CAD build for the part. Positions are in the model's coordinates, mm. Face numbers are marked on the shaded views. A direction names the side the tool comes from. Round coordinates to 2 decimals unless told otherwise and drop trailing zeros. Write each loop counter-clockwise with the first axis right and the second up, starting at its lowest first coordinate (ties: lowest second). Pieces come first, ordered by that corner, then holes. Notation, with made-up numbers: (2, 37) - (16, 37) arc R31 ccw to (16, 64) - close; hole circle Ø5 at (83.5, 25). An arc over 180 degrees is marked (long way). Use one line per item in the form item = value. Start each with the question number.
Item 1: Band-saw the part on A-A, the plane x = -2. List the corners of the cut face in (y, z), and give its area (3 significant figures).
Item 2: Drill centre lines: L1, parallel to X at y = 7, z = 182; L2, parallel to X at y = 7.5, z = 60.5; L3, parallel to X at y = -22, z = -4. Where is each one in solid material? Low to high.
Item 3: Band-saw the part on C-C, the plane x = 38. List the corners of the cut face in (y, z), and give its area (3 significant figures).
Item 4: Pin check, flat tips, straight feed: pin 1 (7 mm diameter, centred on x = 38, y = -22.5, fed in from -Z); pin 2 (2 mm diameter, centred on x = 27.5, z = 156.5, fed in from -Y); pin 3 (10 mm diameter, centred on x = -24.5, z = 52.5, fed in from +Y); pin 4 (12.5 mm diameter, centred on y = 4, z = 44.5, fed in from -X). Stop position of each tip, or through.
Item 5: Tool access for the marked faces 1, 2, 3 and 4: list every direction of +Z, -Z, +X, -X, +Y, -Y with a clear straight run to the whole face (end or side of a thin tool).
Item 6: Pull direction Z, two halves, no side cores. Call the marked faces 5, 6, 7 and 8: +Z half, -Z half, draft (parallel to the pull), parting line (faces both ways), or undercut.
Item 7: Band-saw the part on B-B, the plane z = 170. List the corners of the cut face in (x, y).
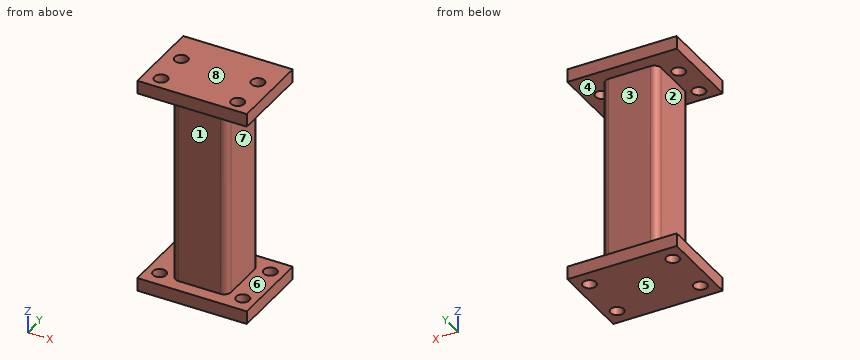
from build123d import *

# Parameters (mm, degrees)
F0_W     = 100
F0_H     = 75
F1_DEPTH = 12
F3_DEPTH = 175.5
F5_W     = 100
F5_H     = 75
F6_DEPTH = 12
F7_D     = 12
F7_DEPTH = 12.001
F9_D     = 12
F9_DEPTH = 12
F9_TIP   = 3.6051637142


with BuildPart() as f1:
    # F0 (on Top) → F1 (new body)
    with BuildSketch(Plane.XY):
        Rectangle(F0_W, F0_H)
    extrude(amount=-F1_DEPTH)

    # F2 (on face) → F3 (join)
    with BuildSketch(Plane.XY):
        with BuildLine():
            Line((-19.05, -25.4), (19.05, -25.4))
            ThreePointArc((19.05, -25.4), (23.5401280605, -23.5401280605), (25.4, -19.05))
            Line((25.4, -19.05), (25.4, 19.05))
            ThreePointArc((25.4, 19.05), (23.5401280605, 23.5401280605), (19.05, 25.4))
            Line((19.05, 25.4), (-19.05, 25.4))
            ThreePointArc((-19.05, 25.4), (-23.5401280605, 23.5401280605), (-25.4, 19.05))
            Line((-25.4, 19.05), (-25.4, -19.05))
            ThreePointArc((-25.4, -19.05), (-23.5401280605, -23.5401280605), (-19.05, -25.4))
        make_face()
        with BuildLine():
            Line((-12.7, 19.05), (12.7, 19.05))
            ThreePointArc((12.7, 19.05), (17.1901280605, 17.1901280605), (19.05, 12.7))
            Line((19.05, 12.7), (19.05, -12.7))
            ThreePointArc((19.05, -12.7), (17.1901280605, -17.1901280605), (12.7, -19.05))
            Line((12.7, -19.05), (-12.7, -19.05))
            ThreePointArc((-12.7, -19.05), (-17.1901280605, -17.1901280605), (-19.05, -12.7))
            Line((-19.05, -12.7), (-19.05, 12.7))
            ThreePointArc((-19.05, 12.7), (-17.1901280605, 17.1901280605), (-12.7, 19.05))
        make_face(mode=Mode.SUBTRACT)
    extrude(amount=F3_DEPTH)

    # F5 (on face) → F6 (join)
    with BuildSketch(Plane.XY.offset(175.5)):
        Rectangle(F5_W, F5_H)
        with BuildLine():
            Line((19.05, -25.4), (-19.05, -25.4))
            ThreePointArc((-19.05, -25.4), (-23.5401280605, -23.5401280605), (-25.4, -19.05))
            Line((-25.4, -19.05), (-25.4, 19.05))
            ThreePointArc((-25.4, 19.05), (-23.5401280605, 23.5401280605), (-19.05, 25.4))
            Line((-19.05, 25.4), (19.05, 25.4))
            ThreePointArc((19.05, 25.4), (23.5401280605, 23.5401280605), (25.4, 19.05))
            Line((25.4, 19.05), (25.4, -19.05))
            ThreePointArc((25.4, -19.05), (23.5401280605, -23.5401280605), (19.05, -25.4))
        make_face(mode=Mode.SUBTRACT)
        with BuildLine():
            ThreePointArc((-25.4, -19.05), (-23.5401280605, -23.5401280605), (-19.05, -25.4))
            Line((-19.05, -25.4), (19.05, -25.4))
            ThreePointArc((19.05, -25.4), (23.5401280605, -23.5401280605), (25.4, -19.05))
            Line((25.4, -19.05), (25.4, 19.05))
            ThreePointArc((25.4, 19.05), (23.5401280605, 23.5401280605), (19.05, 25.4))
            Line((19.05, 25.4), (-19.05, 25.4))
            ThreePointArc((-19.05, 25.4), (-23.5401280605, 23.5401280605), (-25.4, 19.05))
            Line((-25.4, 19.05), (-25.4, -19.05))
        make_face()
        with BuildLine():
            Line((-19.05, -12.7), (-19.05, 12.7))
            ThreePointArc((-19.05, 12.7), (-17.1901280605, 17.1901280605), (-12.7, 19.05))
            Line((-12.7, 19.05), (12.7, 19.05))
            ThreePointArc((12.7, 19.05), (17.1901280605, 17.1901280605), (19.05, 12.7))
            Line((19.05, 12.7), (19.05, -12.7))
            ThreePointArc((19.05, -12.7), (17.1901280605, -17.1901280605), (12.7, -19.05))
            Line((12.7, -19.05), (-12.7, -19.05))
            ThreePointArc((-12.7, -19.05), (-17.1901280605, -17.1901280605), (-19.05, -12.7))
        make_face(mode=Mode.SUBTRACT)
        with BuildLine():
            ThreePointArc((-12.7, 19.05), (-17.1901280605, 17.1901280605), (-19.05, 12.7))
            Line((-19.05, 12.7), (-19.05, -12.7))
            ThreePointArc((-19.05, -12.7), (-17.1901280605, -17.1901280605), (-12.7, -19.05))
            Line((-12.7, -19.05), (12.7, -19.05))
            ThreePointArc((12.7, -19.05), (17.1901280605, -17.1901280605), (19.05, -12.7))
            Line((19.05, -12.7), (19.05, 12.7))
            ThreePointArc((19.05, 12.7), (17.1901280605, 17.1901280605), (12.7, 19.05))
            Line((12.7, 19.05), (-12.7, 19.05))
        make_face()
    extrude(amount=F6_DEPTH)

    # F7 (through all, one way)
    with BuildSketch(Plane.XY):
        with Locations((-38, 22.5), (38, 22.5), (38, -22.5), (-38, -22.5)):
            Circle(F7_D / 2)
    extrude(amount=-F7_DEPTH, mode=Mode.SUBTRACT)

    # F9
    with Locations(Plane.XY.offset(187.5)):
        with Locations((-35, 7.5), (-35, -25.5), (35, -25.5), (35, 7.5)):
            Hole(F9_D / 2, depth=F9_DEPTH)
            with Locations((0, 0, -(F9_DEPTH + F9_TIP / 2))):  # 118° drill point
                Cone(0, F9_D / 2, F9_TIP, mode=Mode.SUBTRACT)


solid = f1.part
Determined:
q1.outline = (-37.5, -12) - (37.5, -12) - (37.5, 0) - (25.4, 0) - (25.4, 175.5) - (37.5, 175.5) - (37.5, 187.5) - (-37.5, 187.5) - (-37.5, 175.5) - (-25.4, 175.5) - (-25.4, 0) - (-37.5, 0) - close; hole (-19.05, 0) - (19.05, 0) - (19.05, 175.5) - (-19.05, 175.5) - close
q1.area = 4,030 mm²
q2.L1 = -50 to -40.98, -29.02 to 29.02, 40.98 to 50
q2.L2 = -25.4 to -19.05, 19.05 to 25.4
q2.L3 = -50 to -43.98, -32.02 to 32.02, 43.98 to 50
q3.outline = (-37.5, -12) - (-28.5, -12) - (-28.5, 0) - (-37.5, 0) - close; (-37.5, 175.5) - (-30.7, 175.5) - (-30.7, 187.5) - (-37.5, 187.5) - close; (-20.3, 175.5) - (2.3, 175.5) - (2.3, 187.5) - (-20.3, 187.5) - close; (-16.5, -12) - (16.5, -12) - (16.5, 0) - (-16.5, 0) - close; (12.7, 175.5) - (37.5, 175.5) - (37.5, 187.5) - (12.7, 187.5) - close; (28.5, -12) - (37.5, -12) - (37.5, 0) - (28.5, 0) - close
q3.area = 1,260 mm²
q4.pin_1 = 175.5
q4.pin_2 = through
q4.pin_3 = 25.38
q4.pin_4 = -25.4
q5.face_1 = +X, -X, -Y
q5.face_2 = -X, +Y, -Y
q5.face_3 = +X, -X, +Y
q5.face_4 = none
q6.face_5 = -Z half
q6.face_6 = undercut
q6.face_7 = undercut
q6.face_8 = +Z half
q7.outline = (-25.4, -19.05) arc R6.35 ccw to (-19.05, -25.4) - (19.05, -25.4) arc R6.35 ccw to (25.4, -19.05) - (25.4, 19.05) arc R6.35 ccw to (19.05, 25.4) - (-19.05, 25.4) arc R6.35 ccw to (-25.4, 19.05) - close; hole (-19.05, -12.7) arc R6.35 ccw to (-12.7, -19.05) - (12.7, -19.05) arc R6.35 ccw to (19.05, -12.7) - (19.05, 12.7) arc R6.35 ccw to (12.7, 19.05) - (-12.7, 19.05) arc R6.35 ccw to (-19.05, 12.7) - close
